from build123d import *

# Parameters (mm, degrees)
SKETCH014_R     = 9
SKETCH014_R_2   = 4
PAD003_DEPTH    = 1.6
SKETCH015_W     = 6.5
SKETCH015_H     = 6
POCKET007_DEPTH = 1.2
POCKET007_TAPER = 40
SKETCH016_R     = 2.65
PAD004_DEPTH    = 4
SKETCH017_R     = 1.25
HOLE001_DEPTH   = 4.2
HOLE001_TIPS_R  = 1.25
PAD005_DEPTH    = 1.3
PAD006_DEPTH    = 6.5
CHAMFER003_SIZE = 0.6
CHAMFER004_SIZE = 1


with BuildPart() as part:
    # Sketch014 → Pad003 (new body)
    with BuildSketch(Plane.XY):
        with BuildLine():
            Line((-30.7, -19.5), (30.7, -19.5))
            ThreePointArc((30.7, -19.5), (50.2, 0), (30.7, 19.5))
            Line((30.7, 19.5), (-30.7, 19.5))
            ThreePointArc((-30.7, 19.5), (-50.2, 0), (-30.7, -19.5))
        make_face()
        Circle(SKETCH014_R, mode=Mode.SUBTRACT)
        with Locations((-13, -13.8)):
            Circle(SKETCH014_R_2, mode=Mode.SUBTRACT)
        with BuildLine():
            ThreePointArc((-24.429009, 8.663375), (-38.920062, -5.15), (-19.711802, 0.492933))
            ThreePointArc((-18.056619, 2.559098), (-19.275002, 1.839074), (-19.711802, 0.492933))
            ThreePointArc((-18.056619, 2.559098), (-15.277568, 8.5), (-21.812065, 9.063722))
            ThreePointArc((-24.429009, 8.663375), (-23.044816, 8.368584), (-21.812065, 9.063722))
        make_face(mode=Mode.SUBTRACT)
        with BuildLine():
            ThreePointArc((24.429009, -8.663375), (38.920062, 5.15), (19.711802, -0.492933))
            ThreePointArc((18.056619, -2.559098), (19.275002, -1.839074), (19.711802, -0.492933))
            ThreePointArc((18.056619, -2.559098), (15.277568, -8.5), (21.812065, -9.063722))
            ThreePointArc((24.429009, -8.663375), (23.044816, -8.368584), (21.812065, -9.063722))
        make_face(mode=Mode.SUBTRACT)
    extrude(amount=PAD003_DEPTH)

    # Sketch015 → Pocket007 (cut)
    with BuildSketch(Plane.XY):
        with Locations((13.25, -14.2)):
            Rectangle(SKETCH015_W, SKETCH015_H)
    extrude(amount=POCKET007_DEPTH, taper=POCKET007_TAPER, mode=Mode.SUBTRACT)

    # Sketch016 → Pad004 (join)
    with BuildSketch(Plane.XY):
        with Locations((-23, 15)):
            Circle(SKETCH016_R)
        with Locations((23, 15)):
            Circle(SKETCH016_R)
        with Locations((23, -15)):
            Circle(SKETCH016_R)
        with Locations((-23, -15)):
            Circle(SKETCH016_R)
    extrude(amount=-PAD004_DEPTH)

    # Sketch017 → Hole001 (cut)
    with BuildSketch(Plane.XY.offset(-4)):
        with Locations((-23, 15)):
            Circle(SKETCH017_R)
        with Locations((23, 15)):
            Circle(SKETCH017_R)
        with Locations((23, -15)):
            Circle(SKETCH017_R)
        with Locations((-23, -15)):
            Circle(SKETCH017_R)
    extrude(amount=HOLE001_DEPTH, mode=Mode.SUBTRACT)

    # Hole001 tips → Hole001 tip 1 section 0
    with BuildSketch(Plane.XY.offset(0.2), mode=Mode.PRIVATE) as hole001_tip_1_s0:
        with Locations((-23, 15)):
            Circle(HOLE001_TIPS_R)
    loft([hole001_tip_1_s0.sketch, Vertex(-23, 15, 0.951076)], mode=Mode.SUBTRACT)

    # Hole001 tips → Hole001 tip 2 section 0
    with BuildSketch(Plane.XY.offset(0.2), mode=Mode.PRIVATE) as hole001_tip_2_s0:
        with Locations((23, 15)):
            Circle(HOLE001_TIPS_R)
    loft([hole001_tip_2_s0.sketch, Vertex(23, 15, 0.951076)], mode=Mode.SUBTRACT)

    # Hole001 tips → Hole001 tip 3 section 0
    with BuildSketch(Plane.XY.offset(0.2), mode=Mode.PRIVATE) as hole001_tip_3_s0:
        with Locations((23, -15)):
            Circle(HOLE001_TIPS_R)
    loft([hole001_tip_3_s0.sketch, Vertex(23, -15, 0.951076)], mode=Mode.SUBTRACT)

    # Hole001 tips → Hole001 tip 4 section 0
    with BuildSketch(Plane.XY.offset(0.2), mode=Mode.PRIVATE) as hole001_tip_4_s0:
        with Locations((-23, -15)):
            Circle(HOLE001_TIPS_R)
    loft([hole001_tip_4_s0.sketch, Vertex(-23, -15, 0.951076)], mode=Mode.SUBTRACT)

    # Sketch018 → Pad005 (join)
    with BuildSketch(Plane.XZ.offset(19.5)):
        Polygon((-13.2, 0), (-10.717394, -4.3), (10.717394, -4.3), (13.2, 0), align=None)
    extrude(amount=-PAD005_DEPTH)

    # Sketch019 → Pad006 (join, symmetric)
    with BuildSketch(Plane.YZ):
        Polygon((-18.2, -3), (-18.2, 0), (-15.2, 0), align=None)
    extrude(amount=PAD006_DEPTH, both=True)

    # Chamfer003
    chamfer003_edges = [part.edges().sort_by_distance(p)[0] for p in [
        (-25.65, -15, -4),
        (-25.65, 15, -4),
        (20.35, 15, -4),
        (20.35, -15, -4),
    ]]
    chamfer(chamfer003_edges, length=CHAMFER003_SIZE)

    # Chamfer004
    chamfer004_edges = [part.edges().sort_by_distance(p)[0] for p in [
        (-50.2, 0, 1.6),
    ]]
    chamfer(chamfer004_edges, length=CHAMFER004_SIZE)


solid = part.part
Input: part model. Units: mm. Frame: model coordinates. A direction names the side the tool comes from. Coordinates: 2 decimals unless noted, no trailing zeros. Loops run counter-clockwise (first coordinate to the right, second up) from the corner with the lowest first, then second, coordinate; pieces in that order, holes last.
(1) Pull-direction query (Y, two-part tool) for faces 5 (the face through (0.1, -16.7, -1.5)), 6 (the face through (-22.328, 16.054, -1.929)), 7 (the face through (-49.355, 0.41, 1.44)); classes: released by +Y, released by -Y, zero draft, split by the parting line, or undercut.
(2) Set-up query: faces 1 (the face through (-19.262, 1.855, 0.789)), 2 (the face through (-6.5, -17, -1)), 3 (the face through (-21.777, -17.351, -1.676)), 4 (the face through (11.94, -18.86, -2.18)). Return all of +Z, -Z, +X, -X, +Y, -Y with unobstructed straight access to the full face (end or side cutting, diameter ignored); none if empty.
(3) Section D-D on x = -27. Return the cut outline in (y, z), then the cut area to 3 significant figures.
(4) Section A-A on z = -1.65. Count the separate pieces of the cut face and the enclosed holes in it, then the cut area to 3 significant figures.
(5) Section B-B on x = 5.5. Return the cut outline in (y, z).
(6) First-contact query: pin 1 Ø3 at (x, z) = (-34.5, 0) entering from +Y; pin 2 Ø13 at (x, y) = (-18.74, 6.5) entering from -Z; pin 3 Ø10.5 at (x, y) = (18.74, -6.5) entering from +Z; pin 4 Ø1 at (x, z) = (-21, -3.5) entering from +Y. Flat tips, straight axial feed; report the tip coordinate or a pass-through.
(7) Material intervals for probe 1 along X at (y, z) = (14, -2.85); probe 2 along Z at (x, y) = (-7, -13.5); probe 3 along Y at (x, z) = (-30.5, 0.05), sorted ascending.
Data:
1. face 5: released by +Y
1. face 6: undercut
1. face 7: split by the parting line
2. face 1: +Z, -Z
2. face 2: -Z, +Y
2. face 3: -Z
2. face 4: -Z, +X, +Y, -Y
3. outline: (-19.5, 0) - (-9.85, 0) - (-9.85, 1.6) - (-18.5, 1.6) - (-19.5, 0.6) - close; (9.85, 0) - (19.5, 0) - (19.5, 0.6) - (18.5, 1.6) - (9.85, 1.6) - close
3. area: 29.9 mm2
4. separate pieces: 5
4. enclosed holes: 4
4. area: 118 mm2
5. outline: (-19.5, -4.3) - (-18.2, -4.3) - (-18.2, -3) - (-15.2, 0) - (-7.12, 0) - (-7.12, 1.6) - (-18.5, 1.6) - (-19.5, 0.6) - close; (7.12, 0) - (19.5, 0) - (19.5, 0.6) - (18.5, 1.6) - (7.12, 1.6) - close
6. pin 1: stops at y = 19.36
6. pin 2: stops at z = 0
6. pin 3: stops at z = 1.6
6. pin 4: stops at y = 17.18
7. probe 1: x = -25.45 to -23.75, -22.25 to -20.55, 20.55 to 22.25, 23.75 to 25.45
7. probe 2: z = 0 to 1.6
7. probe 3: y = -19.5 to -10.29, 10.29 to 19.5
